Verification items for the finished model (mm, model axes). Round coordinates to 2 decimals unless told otherwise and drop trailing zeros. Order: outer loops, then holes, each group sorted by start corner. A loop starts at its lowest first (then second) coordinate and runs counter-clockwise, first axis right, second up. Notation, with made-up numbers: (15.5, 65.25) -> (54.5, 65.25) arc R34 cw to (54.5, 97.25) -> close; hole circle Ø7 at (13, 37). An arc over 180 degrees is marked (long way). Put each result on its own line as item: value.
```python
from build123d import *

# Parameters (mm, degrees)
ESQUISSE1_W        = 600
ESQUISSE1_H        = 50
BOSS_EXTRU_1_DEPTH = 30
BOSS_EXTRU_2_DEPTH = 10
CHANFREIN1_SIZE    = 2
BOSS_EXTRU_3_DEPTH = 10
CHANFREIN2_SIZE    = 2


with BuildPart() as part:
    # Esquisse1 → Boss.-Extru.1 (new body)
    with BuildSketch(Plane.XY):
        Rectangle(ESQUISSE1_W, ESQUISSE1_H)
    extrude(amount=BOSS_EXTRU_1_DEPTH)

    # Esquisse2 → Boss.-Extru.2 (add)
    with BuildSketch(Plane(origin=(300, 0, 0), x_dir=(0, 0, -1), z_dir=(1, 0, 0))):
        with BuildLine():
            Line((-9, 10), (-9, -10))
            ThreePointArc((-9, -10), (-15, -16), (-21, -10))
            Line((-21, -10), (-21, 10))
            ThreePointArc((-21, 10), (-15, 16), (-9, 10))
        make_face()
    extrude(amount=BOSS_EXTRU_2_DEPTH)

    # Chanfrein1
    chanfrein1_edges = [part.edges().sort_by_distance(p)[0] for p in [
        (310, 16, 15),
        (310, 0, 21),
        (310, -16, 15),
        (310, 0, 9),
    ]]
    chamfer(chanfrein1_edges, length=CHANFREIN1_SIZE)

    # Esquisse3 → Boss.-Extru.3 (add)
    with BuildSketch(Plane.ZY.offset(300)):
        with BuildLine():
            Line((21, 10), (21, -10))
            ThreePointArc((21, -10), (15, -16), (9, -10))
            Line((9, -10), (9, 10))
            ThreePointArc((9, 10), (15, 16), (21, 10))
        make_face()
    extrude(amount=BOSS_EXTRU_3_DEPTH)

    # Chanfrein2
    chanfrein2_edges = [part.edges().sort_by_distance(p)[0] for p in [
        (-310, 0, 21),
        (-310, 16, 15),
        (-310, 0, 9),
        (-310, -16, 15),
    ]]
    chamfer(chanfrein2_edges, length=CHANFREIN2_SIZE)


solid = part.part
```
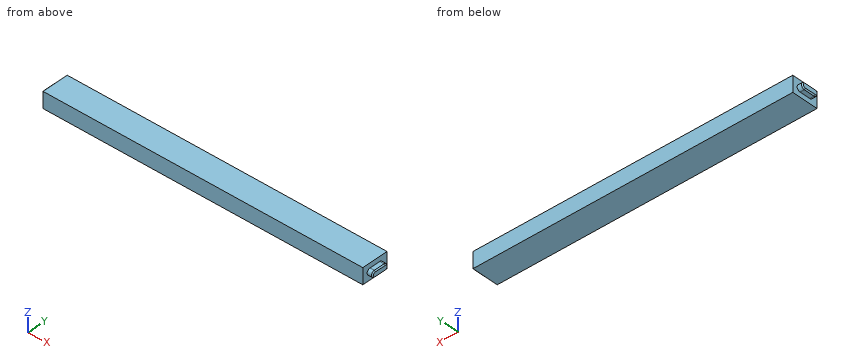
Item 1: Depth check by flat-ended pin: pin 1 Ø4 at (x, y) = (-304.5, 2.5) entering from +Z; pin 2 Ø12 at (y, z) = (19, 10.5) entering from -X; pin 3 Ø4 at (x, y) = (-303, -0.5) entering from -Z. Enter the tip coordinate at first touch or a pass-through.
Geometry check:
pin 1: z = 21
pin 2: x = -309.94
pin 3: z = 9
Item 2: Material ranges on line 1 along X through (y, z) = (9, 22.5), recorded low to high.
Geometry check:
line 1: -300 to 300
Item 3: Sectioned sample at A-A, the plane y = 0. Record the boundary of the cut face in (x, z), then the cut area to 3 significant figures.
Geometry check:
outline: (-310, 11) -> (-308, 9) -> (-300, 9) -> (-300, 0) -> (300, 0) -> (300, 9) -> (308, 9) -> (310, 11) -> (310, 19) -> (308, 21) -> (300, 21) -> (300, 30) -> (-300, 30) -> (-300, 21) -> (-308, 21) -> (-310, 19) -> close
area: 18,200 mm2
